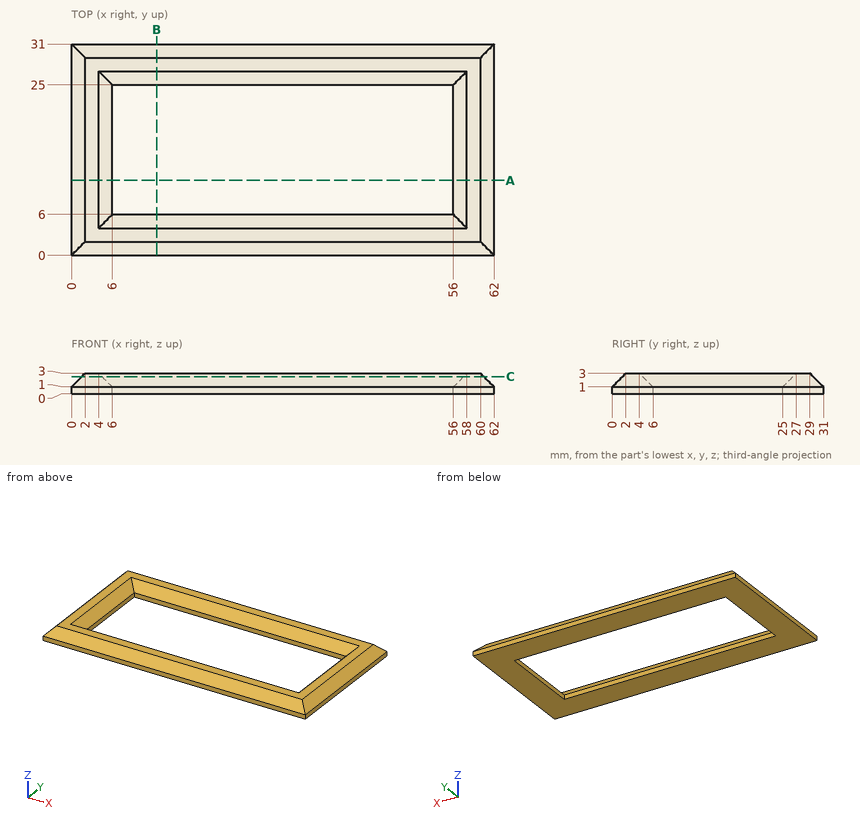
The figure shows three views and two pictorial views of one solid part (mm, origin at its lowest corner). Answer the questions. Round coordinates to 2 decimals unless told otherwise and drop trailing zeros. Order: outer loops, then holes, each group sorted by start corner. A loop starts at its lowest first (then second) coordinate and runs counter-clockwise, first axis right, second up. Notation, with made-up numbers: (76.5, -36.5) -> (91.5, -36.5) arc R34 cw to (91.5, -4.5) -> close; hole circle Ø11 at (-5.75, -4). An arc over 180 degrees is marked (long way). One line per item, written item: value.
Item 1: Find section B-B, the plane x = 12.5. Give the vertices of the cut face in (y, z), then the cut area to 3 significant figures.
Taken from the geometry:
outline: (0, 0) -> (6, 0) -> (6, 1) -> (4, 3) -> (2, 3) -> (0, 1) -> close; (25, 0) -> (31, 0) -> (31, 1) -> (29, 3) -> (27, 3) -> (25, 1) -> close
area: 28.0 mm2
Item 2: Find section A-A, the plane y = 11. Give the vertices of the cut face in (x, z).
Taken from the geometry:
outline: (0, 0) -> (6, 0) -> (6, 1) -> (4, 3) -> (2, 3) -> (0, 1) -> close; (56, 0) -> (62, 0) -> (62, 1) -> (60, 3) -> (58, 3) -> (56, 1) -> close
Item 3: Straight lines are drawn through the part: L1, parallel to Y at x = 17, z = 0.5; L2, parallel to X at y = 20, z = 0.35; L3, parallel to X at y = 9.5, z = 1.7. For each, find the intervals that lie inside material, in ascending order.
Taken from the geometry:
L1: y = 0 to 6, 25 to 31
L2: x = 0 to 6, 56 to 62
L3: x = 0.7 to 5.3, 56.7 to 61.3
Item 4: Given P1, Ø1.5, axis at x = 54, z = 2.5, coming from the -Y side, flat-ended and moving along its own axis, determine where the tip first touches the part or whether it passes through.
Taken from the geometry:
P1: stops at y = 0.75
Item 5: Find section C-C, the plane z = 2.5. Give the vertices of the cut face in (x, y), then the cut area to 3 significant figures.
Taken from the geometry:
outline: (1.5, 1.5) -> (60.5, 1.5) -> (60.5, 29.5) -> (1.5, 29.5) -> close; hole (4.5, 4.5) -> (57.5, 4.5) -> (57.5, 26.5) -> (4.5, 26.5) -> close
area: 486 mm2
